```python
from build123d import *

# Parameters (mm, degrees)
SKETCH4_W           = 23.01079085
SKETCH4_H           = 12.035429775
BOSS_EXTRUDE1_DEPTH = 5


with BuildPart() as part:
    # Sketch4 → Boss-Extrude1 (new body)
    with BuildSketch(Plane.XY):
        with BuildLine():
            Line((-23.029498644, -9.969527596), (0.020059035, -9.969527596))
            ThreePointArc((0.020059035, -9.969527596), (7.083752781, -7.043649902), (10.009630666, 0.020043765))
            Line((10.009630666, 0.020043765), (10.009630666, 12.035429505))
            ThreePointArc((10.009630666, 12.035429505), (7.077737043, 19.110165135), (0.00232147, 22.0404175))
            ThreePointArc((0.00232147, 22.0404175), (-3.734235721, 25.776974691), (0.00232147, 29.513531883))
            Line((0.00232147, 29.513531883), (10.009630666, 31.965921786))
            ThreePointArc((10.009630666, 31.965921786), (6.784699168, 36.172527862), (1.631535857, 37.413747311))
            ThreePointArc((1.631535857, 37.413747311), (-76.612020645, 26.532654718), (-152.922807067, 6.10923224))
            ThreePointArc((-152.922807067, 6.10923224), (-155.131459045, 5.328115377), (-157.265351369, 4.361269649))
            ThreePointArc((-157.265351369, 4.361269649), (-158.533663589, 0.498259669), (-154.67065361, -0.770052551))
            ThreePointArc((-154.67065361, -0.770052551), (-153.805456008, -0.356328461), (-152.922807067, 0.018725346))
            ThreePointArc((-152.922807067, 0.018725346), (-93.417009782, 10.900895291), (-33.017751587, 14.261124841))
            Line((-33.017751587, 14.261124841), (-33.017751587, 12.035429775))
            Line((-33.017751587, 12.035429775), (-33.017751587, 0.018725346))
            ThreePointArc((-33.017751587, 0.018725346), (-30.092260032, -7.044036042), (-23.029498644, -9.969527596))
        make_face()
        with Locations((-11.505395425, 6.017714888)):
            Rectangle(SKETCH4_W, SKETCH4_H, mode=Mode.SUBTRACT)
    extrude(amount=BOSS_EXTRUDE1_DEPTH)


solid = part.part
```
Input: part model. Units: mm. Frame: model coordinates. A direction names the side the tool comes from. Round coordinates to 2 decimals unless told otherwise and drop trailing zeros. Loops run counter-clockwise (first coordinate to the right, second up) from the corner with the lowest first, then second, coordinate; pieces in that order, holes last. Notation, with made-up numbers: (69.5, 8) -> (77.5, 8) arc R22 cw to (77.5, 34) -> close; hole circle Ø7 at (86, 19.5). An arc over 180 degrees is marked (long way). Write each question's results on one line, items separated by ' | '.
1. Section A-A (z = 4.05). Return loops of the section in (x, y).
Geometry results:
outline: (-157.27, 4.36) arc R2.88 ccw to (-154.67, -0.77) arc R21.68 cw to (-152.92, 0.02) arc R483.1 cw to (-33.02, 14.26) -> (-33.02, 0.02) arc R9.99 ccw to (-23.03, -9.97) -> (0.02, -9.97) arc R9.99 ccw to (10.01, 0.02) -> (10.01, 12.04) arc R10.01 ccw to (0, 22.04) arc R3.74 cw to (0, 29.51) -> (10.01, 31.97) arc R7.94 ccw to (1.63, 37.41) arc R640.96 ccw to (-152.92, 6.11) arc R27.41 ccw to start; hole (-23.01, 0) -> (0, 0) -> (0, 12.04) -> (-23.01, 12.04) -> close
2. First-contact query: P1, Ø2.5, axis at y = 6, z = 2, coming from the -X side; P2, Ø1, axis at x = -91, z = 3.5, coming from the -Y side. Flat tips, straight axial feed; report the tip coordinate or a pass-through.
Geometry results:
P1: x = -156.46 | P2: y = 11.12
3. Ray query, line 1 (Y direction, x = -15, z = 2.45); line 2 (Y direction, x = 0.5, z = 3.8); line 3 (Y direction, x = -66.5, z = 4.2). Return the intervals inside material, ascending. Write a range as from..to.
Geometry results:
line 1: -9.97..0, 12.04..35.92 | line 2: -9.96..22.03, 29.64..37.33 | line 3: 13.34..28.5
4. Set-up query: faces 1 (the face through (-50, 16, 5)), 2 (the face through (-12, 12.035, 2)), 3 (the face through (7.155, 19.032, 2.465)). Return all of +Z, -Z, +X, -X, +Y, -Y with unobstructed straight access to the full face (end or side cutting, diameter ignored); none if empty.
Geometry results:
face 1: +Z, +X, -X, +Y, -Y | face 2: +Z, -Z | face 3: +Z, -Z, +X
5. Section D-D (y = 26). Return loops of the section in (x, z), and give its area (3 significant figures).
Geometry results:
outline: (-79.21, 0) -> (-3.73, 0) -> (-3.73, 5) -> (-79.21, 5) -> close | area: 377 mm2
6. Mould query, pull axis X, two halves, no side actions, for faces 4 (the face through (-3.733, 25.695, 2.465)), 5 (the face through (-75.53, 26.75, 2.46)), 6 (the face through (-94.26, 10.8, 2.46)). Classes: +X half, -X half, draft (parallel to the pull), parting line (faces both ways), or undercut.
Geometry results:
face 4: +X half | face 5: -X half | face 6: undercut
7. Section B-B (y = 9.5). Return loops of the section in (x, z).
Geometry results:
outline: (-142.5, 0) -> (-104.18, 0) -> (-104.18, 5) -> (-142.5, 5) -> close; (-33.02, 0) -> (-23.01, 0) -> (-23.01, 5) -> (-33.02, 5) -> close; (0, 0) -> (10.01, 0) -> (10.01, 5) -> (0, 5) -> close
8. Section C-C (x = -138). Return loops of the section in (y, z), and give its area (3 significant figures).
Geometry results:
outline: (3.48, 0) -> (10.9, 0) -> (10.9, 5) -> (3.48, 5) -> close | area: 37.1 mm2
